Check sheet for the drawn part. Datum: minimum x, y, z corner. Units: mm. Round coordinates to 2 decimals unless told otherwise and drop trailing zeros. Write each loop counter-clockwise with the first axis right and the second up, starting at its lowest first coordinate (ties: lowest second). Pieces come first, ordered by that corner, then holes. Notation, with made-up numbers: M 59.5,77 L 115.5,77 A30 cw 115.5,109 Z; hole C -1.5,46 d2. An arc over 180 degrees is marked long. Put each result on its own line as item: value.
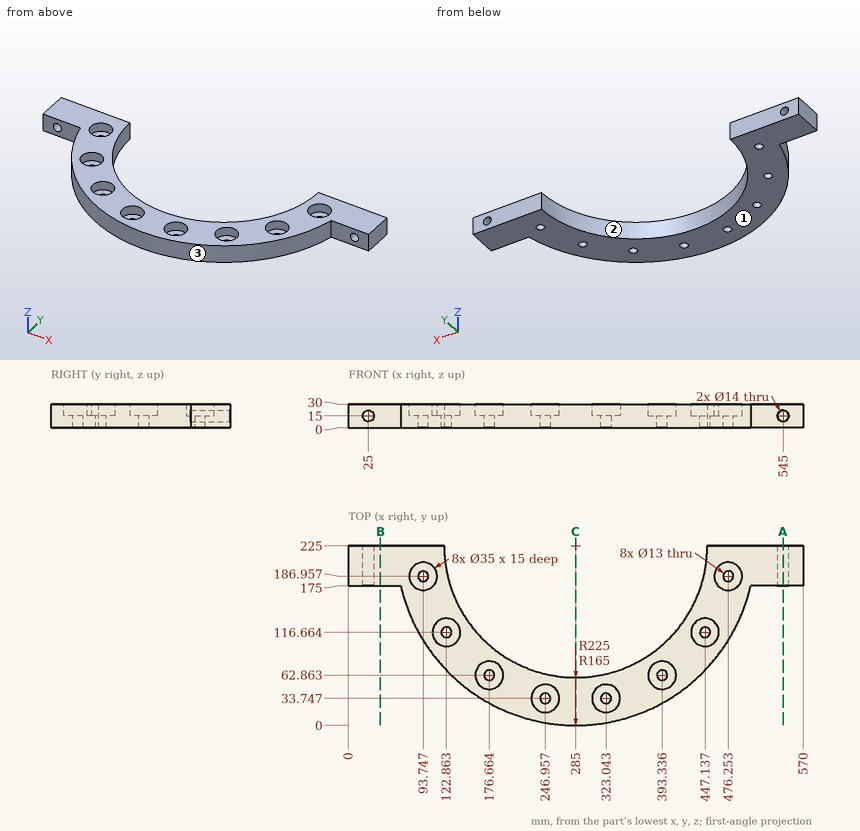
1. Cross-section at B-B (x = 40). Enter the section's corners in (y, z), then the cut area to 3 significant figures.
Computed values:
outline: M 175,0 L 225,0 L 225,30 L 175,30 Z
area: 1,500 mm2
2. Depth check by flat-ended pin: pin 1 Ø1.5 at (x, y) = (117.5, 92.5) entering from -Z; pin 2 Ø17 at (x, y) = (93.75, 186.96) entering from +Z; pin 3 Ø3 at (y, z) = (169, 11) entering from +X; pin 4 Ø6 at (y, z) = (141, 6.5) entering from -X (1 decimal). Enter the tip coordinate at first touch or a pass-through.
Computed values:
pin 1: stops at z = 0
pin 2: stops at z = 15
pin 3: stops at x = 503.3
pin 4: stops at x = 75.1
3. Cross-section at A-A (x = 545). Enter the section's corners in (y, z), then the cut area to 3 significant figures.
Computed values:
outline: M 175,0 L 225,0 L 225,8 L 175,8 Z; M 175,22 L 225,22 L 225,30 L 175,30 Z
area: 800 mm2
4. Cross-section at C-C (x = 285). Enter the section's corners in (y, z).
Computed values:
outline: M 0,0 L 60,0 L 60,30 L 0,30 Z
5. Scan lines: probe 1 along X at (y, z) = (74.5, 23) (1 decimal); probe 2 along X at (y, z) = (59, 4.25) (1 decimal); probe 3 along Y at (x, z) = (280, 27.25) (1 decimal). Record each from-to range of solid material in increasing order.
Computed values:
probe 1: x = 117.7 to 163.6, 189.7 to 217.4, 352.6 to 380.3, 406.4 to 452.3
probe 2: x = 133.1 to 171.4, 181.9 to 388.1, 398.6 to 436.9
probe 3: y = 0.1 to 60.1
6. Release check for a two-part mould opening along X. For the marked faces 1, 2 and 3 record: +X half, -X half, draft (parallel to the pull), parting line (faces both ways), or undercut.
Computed values:
face 1: draft
face 2: undercut
face 3: parting line
